Can you work these out from the drawing? Everything is in mm from the part's minimum corner. Give positions to 0.01 mm unless a question says otherwise; leave off trailing zeros. Loops run counter-clockwise (first coordinate to the right, second up) from the corner with the lowest first, then second, coordinate; pieces in that order, holes last. Notation, with made-up numbers: (73.25, 52) - (113.25, 52) arc R15 ccw to (113.25, 59) - close; hole circle Ø3 at (5.25, 22). An arc over 180 degrees is marked (long way). One line per item, written item: value. Start each with the question number.
Q1. I want a section at A-A (x = 35). Please give me the cut outline in (y, z).
Q2. I want a section at B-B (y = 47). Please give me the cut outline in (x, z) (1 decimal).
Q3. I want a section at D-D (z = 2.75). Count the separate pieces of the cut face and the enclosed holes in it, then the cut area to 3 significant figures.
Q4. I'm going to push flat-ended pins straight in: P1, Ø2, axis at x = 56, y = 22.5, coming from the +Z side; P2, Ø3, axis at y = 12.5, z = 3, coming from the -X side; P3, Ø2, axis at x = 53.5, z = 4, coming from the +Y side; P4, Ø6, axis at x = 35, y = 59, coming from the +Z side. Where does each tip first touch, or does it pass through?
Q5. If I drill on line 1 (Y direction, x = 13.5, z = 0.75); line 2 (Y direction, x = 15, z = 6.75) (1 decimal); line 3 (X direction, y = 11, z = 7.3) (1 decimal), over which ranges is the centre line in solid material (lowest first)? Write a range as from..to.
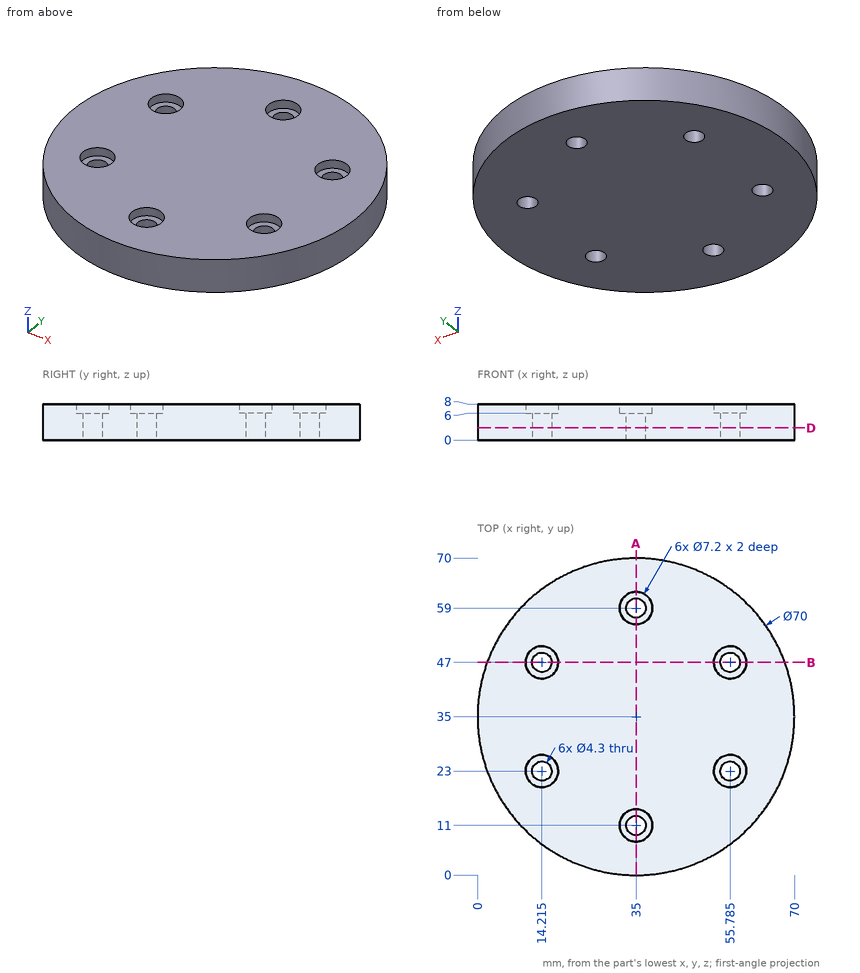
Worked answers:
1. outline: (0, 0) - (8.85, 0) - (8.85, 6) - (7.4, 6) - (7.4, 8) - (0, 8) - close; (13.15, 0) - (56.85, 0) - (56.85, 6) - (55.4, 6) - (55.4, 8) - (14.6, 8) - (14.6, 6) - (13.15, 6) - close; (61.15, 0) - (70, 0) - (70, 8) - (62.6, 8) - (62.6, 6) - (61.15, 6) - close
2. outline: (2.1, 0) - (12.1, 0) - (12.1, 6) - (10.6, 6) - (10.6, 8) - (2.1, 8) - close; (16.4, 0) - (53.6, 0) - (53.6, 6) - (52.2, 6) - (52.2, 8) - (17.8, 8) - (17.8, 6) - (16.4, 6) - close; (57.9, 0) - (67.9, 0) - (67.9, 8) - (59.4, 8) - (59.4, 6) - (57.9, 6) - close
3. separate pieces: 1
3. enclosed holes: 6
3. area: 3,760 mm²
4. P1: passes through
4. P2: stops at x = 7
4. P3: stops at y = 65.31
4. P4: stops at z = 6
5. line 1: y = 7.38..20.97, 25.03..44.97, 49.03..62.62
5. line 2: y = 6.3..19.5, 26.5..43.5, 50.5..63.7
5. line 3: x = 9.5..31.4, 38.6..60.5
